Answer from the drawing. Dimensions are ordinates in mm from the lowest x, y and z of the part. Give positions to 0.01 mm unless a question says otherwise; leave off trailing zeros. Write each loop counter-clockwise with the first axis right and the second up, starting at its lowest first coordinate (ties: lowest second). Pieces come first, ordered by that corner, then holes.
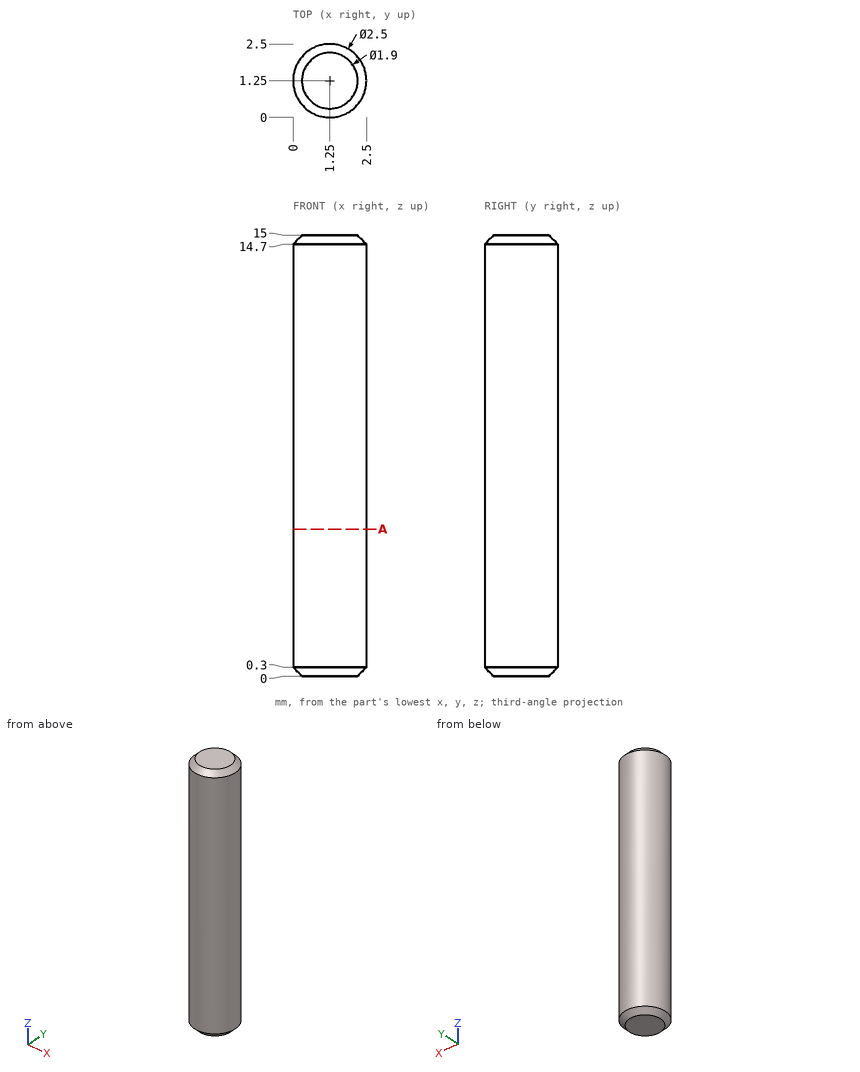
Item 1: This flat-tipped pin is pushed along its axis until it touches: P1, Ø1, axis at y = 1.5, z = 8, coming from the -X side. Where does it stop, or does it pass through?
Conclusion:
P1: stops at x = 0
Item 2: Consider probe 1 along Y at (x, z) = (1.3, 7.5); probe 2 along X at (y, z) = (1.4, 10); probe 3 along Y at (x, z) = (2.3, 6.75). Determine where each line is inside the solid, lowest interval first.
Conclusion:
probe 1: y = 0 to 2.5
probe 2: x = 0.01 to 2.49
probe 3: y = 0.57 to 1.93
Item 3: A cutting plane is placed at A-A, the plane z = 5. Give the vertices of the cut face in (x, y).
Conclusion:
outline: circle Ø2.5 at (1.25, 1.25)
